Read the model definition and answer for the solid it produces. Units are mm, in the model's axes. Give positions to 0.01 mm unless a question says otherwise; leave off trailing zeros. Write each loop counter-clockwise with the first axis right and the second up, starting at its lowest first coordinate (ties: lowest second). Pieces come first, ordered by that corner, then holes. Notation, with made-up numbers: (15, 58) -> (58, 58) arc R22 cw to (58, 70) -> close; hole circle Ø2 at (-31.5, 50). An arc over 180 degrees is marked (long way). Use a Markdown table: item, result.
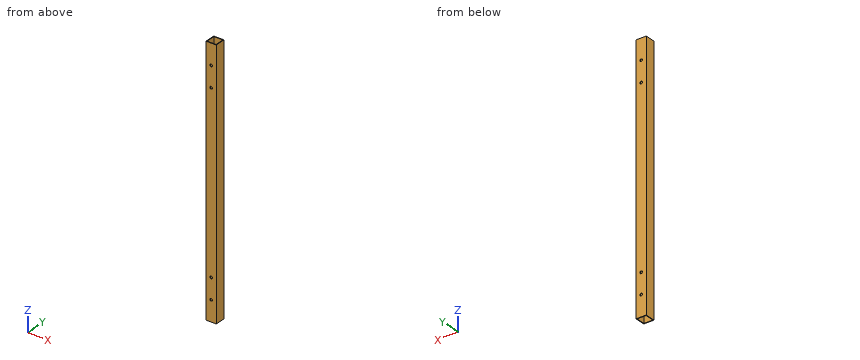
Autodesk Inventor part; units mm, degrees
ref_plane "YZ Plane" through (0, 0, 0) normal (1, 0, 0) x (0, 1, 0)
ref_plane "XZ Plane" through (0, 0, 0) normal (0, 1, 0) x (-1, 0, 0)
ref_plane "XY Plane" through (0, 0, 0) normal (0, 0, 1) x (1, 0, 0)
sketch "Sketch1" plane through (0, 0, 0) normal (0, 0, 1) x (1, 0, 0)
  line L0 (0, 0) -> (25.4, 0)
  line L1 (25.4, 0) -> (25.4, 25.4)
  line L2 (25.4, 25.4) -> (0, 25.4)
  line L3 (0, 25.4) -> (0, 0)
  dimension "d0" = 25.4
  dimension "d1" = 25.4
extrude "Extrusion1" add sketch "Sketch1" along normal blind 635
shell "Shell1" thickness 1.5875 removed faces 2 at (8.4667, 16.9333, 0) at (16.9333, 8.4667, 635)
sketch "Sketch2" plane through (0, 25.4, 0) normal (0, 1, 0) x (1, 0, 0)
  line L0 (0, -635) -> (25.4, -635)
  line L1 (25.4, 0) -> (0, 0)
  line L2 (0, 0) -> (0, -635)
  circle A0 centre (12.7, -50.8) radius 3.175
  circle A1 centre (12.7, -101.6) radius 3.175
  circle A2 centre (12.7, -533.4) radius 3.175
  circle A3 centre (12.7, -584.2) radius 3.175
  dimension "d7" = 50.8
  dimension "d8" = 50.8
  dimension "d9" = 12.7
  dimension "d10" = 12.7
  dimension "d11" = 6.35
  dimension "d12" = 6.35
  dimension "d13" = 12.7
  dimension "d14" = 12.7
  dimension "d15" = 50.8
  dimension "d16" = 50.8
  dimension "d17" = 6.35
  dimension "d18" = 6.35
extrude "Extrusion2" cut sketch "Sketch2" against normal through all
properties part number "DriveTrain_SideRail" material "Aluminum-6061"
Item 1: This flat-tipped pin is pushed along its axis until it touches: P1, Ø8, axis at x = 6.5, y = 19.5, coming from the +Z side. Where does it stop, or does it pass through?
Return value:
| item | result |
|---|---|
| P1 | through |
Item 2: A cutting plane is placed at B-B (y = 19.75). Give the vertices of the cut face in (x, z).
Return value:
| item | result |
|---|---|
| outline | (0, 0) -> (1.59, 0) -> (1.59, 635) -> (0, 635) -> close; (23.81, 0) -> (25.4, 0) -> (25.4, 635) -> (23.81, 635) -> close |
Item 3: Straight lines are drawn through the part: line 1 along Z through (x, y) = (12.7, 24.3) (3 decimals); line 2 along Y through (x, z) = (8, 43.5); line 3 along X through (y, z) = (24.9, 50.8) (3 decimals). For each, find the intervals that lie inside material, in ascending order. Write a range as [from, to].
Return value:
| item | result |
|---|---|
| line 1 | [0, 47.625], [53.975, 98.425], [104.775, 530.225], [536.575, 581.025], [587.375, 635] |
| line 2 | [0, 1.59], [23.81, 25.4] |
| line 3 | [0, 9.525], [15.875, 25.4] |
Item 4: A cutting plane is placed at A-A (z = 217.5). Give the vertices of the cut face in (x, y).
Return value:
| item | result |
|---|---|
| outline | (0, 0) -> (25.4, 0) -> (25.4, 25.4) -> (0, 25.4) -> close; hole (1.59, 1.59) -> (23.81, 1.59) -> (23.81, 23.81) -> (1.59, 23.81) -> close |
